Can you work these out from the model? Positions are in its coordinate system, mm. Face numbers are marked on the shaded views. A direction names the side the tool comes from. Give positions to 0.01 mm unless a question says otherwise; leave off trailing zeros. Loops run counter-clockwise (first coordinate to the right, second up) from the corner with the lowest first, then second, coordinate; pieces in that order, holes last. Notation, with made-up numbers: (6, -31.5) -> (21, -31.5) arc R8 cw to (21, -26.5) -> close; hole circle Ø2 at (45.25, 47.25). An arc over 180 degrees is marked (long way). Use CSV: the item, a comma, the result in double quotes.
from build123d import *

# Parameters (mm, degrees)
F0_W      = 60
F0_H      = 40
F1_DEPTH  = 50
F3_R      = 35
F4_DEPTH  = 10
F6_DEPTH  = 10
F7_W      = 20
F7_H      = 10
F8_DEPTH  = 60
F10_DEPTH = 50.001
F12_DEPTH = 25
F14_DEPTH = 25


with BuildPart() as f1:
    # F0 (on Top) → F1 (new body)
    with BuildSketch(Plane.XY):
        with Locations((-8.7906960398, 1.5665522108)):
            Rectangle(F0_W, F0_H)
    extrude(amount=F1_DEPTH)

    # F3 (on offset) → F4 (cut)
    with BuildSketch(Plane(origin=(-28.7906960398, 0, 0), x_dir=(0, -1, 0), z_dir=(-1, 0, 0))):
        with Locations((18.4334477892, 50)):
            Circle(F3_R)
    extrude(amount=-F4_DEPTH, mode=Mode.SUBTRACT)

    # F5 (on face) → F6 (cut)
    with BuildSketch(Plane(origin=(-38.7906960398, 0, 0), x_dir=(0, -1, 0), z_dir=(-1, 0, 0))):
        Polygon((18.4334477892, 50), (-1.5665522108, 50), (18.4334477892, 40), align=None)
    extrude(amount=-F6_DEPTH, mode=Mode.SUBTRACT)

    # F7 (on face) → F8 (cut, through all)
    with BuildSketch(Plane.YZ.offset(21.2093039602)):
        with Locations((1.5665522108, 5)):
            Rectangle(F7_W, F7_H)
    extrude(amount=-F8_DEPTH, mode=Mode.SUBTRACT)

    # F9 (on face) → F10 (cut, through all)
    with BuildSketch(Plane.XY.offset(50)):
        Polygon((21.2093039602, -18.4334477892), (21.2093039602, 11.5665522108), (6.2093039602, 1.5665522108), (-8.7906960398, -18.4334477892), align=None)
    extrude(amount=-F10_DEPTH, mode=Mode.SUBTRACT)

    # F11 (on face) → F12 (cut)
    with BuildSketch(Plane(origin=(0, 21.5665522108, 0), x_dir=(-1, 0, 0), z_dir=(0, 1, 0))):
        Polygon((-6.2093039602, 50), (-21.2093039602, 50), (-21.2093039602, 10), align=None)
    extrude(amount=-F12_DEPTH, mode=Mode.SUBTRACT)

    # F13 (on face) → F14 (cut)
    with BuildSketch(Plane(origin=(-18.7906960398, 0, 0), x_dir=(0, -1, 0), z_dir=(-1, 0, 0))):
        Polygon((18.4334477892, 50), (-1.5665522108, 50), (18.4334477892, 30), align=None)
    extrude(amount=-F14_DEPTH, mode=Mode.SUBTRACT)


solid = f1.part
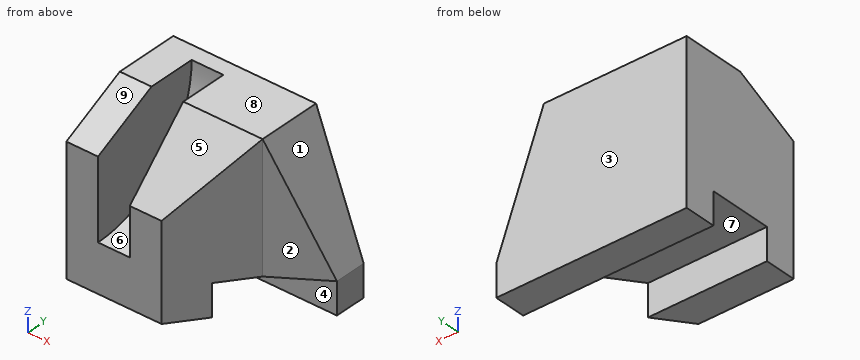
(1) If I drill on L1, parallel to Y at x = -11.5, z = 7.5; L2, parallel to X at y = 2, z = 34.5; L3, parallel to X at y = 11.5, z = 34.5, over which ranges is the centre line in solid material (lowest first)? Write a range as from..to.
Answer sheet:
L1,"y = -18.43..-8.43, 11.57..21.57"
L2,"x = -38.79..-28.79, -18.79..6.86"
L3,"x = -38.79..-28.79, -18.79..12.02"
(2) If we section it at A-A, the plane z = 7: Write out the boundary of the cut face in (x, y), then the cut area to 4 significant figures.
Answer sheet:
outline,"(-38.79, -18.43) -> (-8.79, -18.43) -> (-1.29, -8.43) -> (-38.79, -8.43) -> close; (-38.79, 11.57) -> (21.21, 11.57) -> (21.21, 21.57) -> (-38.79, 21.57) -> close"
area,"937.5 mm2"
(3) Will these pins go through, and if not, where does the flat tip stop? pin 1 Ø10 at (x, y) = (-19, -6) entering from +Z; pin 2 Ø6 at (x, z) = (9, 39) entering from -Y; pin 3 Ø6 at (x, z) = (-1, 33) entering from -Y.
Answer sheet:
pin 1,"stops at z = 47.43"
pin 2,"stops at y = 1.29"
pin 3,"stops at y = -12.05"
(4) If we section it at B-B, the plane x = -11: Write out the boundary of the cut face in (y, z), then the cut area to 3 significant figures.
Answer sheet:
outline,"(-18.43, 0) -> (-8.43, 0) -> (-8.43, 10) -> (11.57, 10) -> (11.57, 0) -> (21.57, 0) -> (21.57, 50) -> (1.57, 50) -> (-18.43, 30) -> close"
area,"1,600 mm2"
(5) Which directions (+Z, -Z, +X, -X, +Y, -Y) give clear straight access to the entire face, cutting with the end or side of a thin tool? Please do the marked faces 5, 6, 7, 8 and 9.
Answer sheet:
face 5,"+Z, +X, -Y"
face 6,"+Z, -Y"
face 7,"-Z, +X, -X"
face 8,"+Z, +X, -X, +Y, -Y"
face 9,"+Z, +X, -X, -Y"
(6) If we section it at D-D, the plane z = 17: Write out the boundary of the cut face in (x, y), then the cut area to 3 significant figures.
Answer sheet:
outline,"(-38.79, -18.43) -> (-28.79, -18.43) -> (-28.79, -6.77) -> (-18.79, -6.77) -> (-18.79, -18.43) -> (-8.79, -18.43) -> (6.21, 1.57) -> (18.58, 9.82) -> (18.58, 21.57) -> (-38.79, 21.57) -> close"
area,"1,730 mm2"
(7) If we section it at C-C, the plane y = 17.5: Write out the boundary of the cut face in (x, z), then the cut area to 3 significant figures.
Answer sheet:
outline,"(-38.79, 0) -> (21.21, 0) -> (21.21, 10) -> (6.21, 50) -> (-38.79, 50) -> close"
area,"2,700 mm2"
(8) We'd pull the mould along Y, two halves only. Please class the marked faces 1, 2, 3 and 4: released by +Y, released by -Y, zero draft, split by the parting line, or undercut.
Answer sheet:
face 1,"zero draft"
face 2,"released by -Y"
face 3,"released by +Y"
face 4,"undercut"
